from build123d import *

# Parameters (mm, degrees)
BOSS_EXTRUDE1_DEPTH = 1.6
SKETCH2_R           = 1.5875
CUT_EXTRUDE1_DEPTH  = 47.534935159


with BuildPart() as part:
    # Sketch1 → Boss-Extrude1 (new body)
    with BuildSketch(Plane(origin=(0, 0, 0), x_dir=(1, 0, 0), z_dir=(0, 1, 0))):
        with BuildLine():
            Line((-23.0632, 31.273950746), (-19.05, 31.273950746))
            ThreePointArc((-19.05, 31.273950746), (-15.214318255, 32.713055735), (-13.055721082, 36.195))
            Line((-13.055721082, 36.195), (-13.055721082, 40.386))
            Line((-13.055721082, 40.386), (13.055721082, 40.386))
            Line((13.055721082, 40.386), (13.055721082, 36.195))
            ThreePointArc((13.055721082, 36.195), (15.214318255, 32.713055735), (19.05, 31.273950746))
            Line((19.05, 31.273950746), (23.0632, 31.273950746))
            Line((23.0632, 31.273950746), (23.0632, -31.273950746))
            Line((23.0632, -31.273950746), (19.05, -31.273950746))
            ThreePointArc((19.05, -31.273950746), (15.214318255, -32.713055735), (13.055721082, -36.195))
            Line((13.055721082, -36.195), (13.055721082, -40.386))
            Line((13.055721082, -40.386), (-13.055721082, -40.386))
            Line((-13.055721082, -40.386), (-13.055721082, -36.195))
            ThreePointArc((-13.055721082, -36.195), (-15.214318255, -32.713055735), (-19.05, -31.273950746))
            Line((-19.05, -31.273950746), (-23.0632, -31.273950746))
            Line((-23.0632, -31.273950746), (-23.0632, 0))
            Line((-23.0632, 0), (-23.0632, 31.273950746))
        make_face()
    extrude(amount=BOSS_EXTRUDE1_DEPTH)

    # Sketch2 → Cut-Extrude1 (cut, through all)
    with BuildSketch(Plane(origin=(0, 1.6, 0), x_dir=(1, 0, 0), z_dir=(0, 1, 0))):
        with Locations(Location((-19.05, 12.7, 0), (0, 0, 270))):
            Circle(SKETCH2_R)
        with Locations(Location((19.05, 12.7, 0), (0, 0, 90))):
            Circle(SKETCH2_R)
        with Locations(Location((19.05, -12.7, 0), (0, 0, 270))):
            Circle(SKETCH2_R)
        with Locations(Location((-19.05, -12.7, 0), (0, 0, 90))):
            Circle(SKETCH2_R)
    extrude(amount=-CUT_EXTRUDE1_DEPTH, mode=Mode.SUBTRACT)


solid = part.part
The model under review builds one solid part; all positions refer to its coordinate system, in mm. A direction names the side the tool comes from. Coordinates: 2 decimals unless noted, no trailing zeros. Loops run counter-clockwise (first coordinate to the right, second up) from the corner with the lowest first, then second, coordinate; pieces in that order, holes last.
(1) Consider section A-A, the plane z = 12.7. Give the boundary of the cut face in (x, y), plus the area to 3 significant figures.
Determined:
outline: (-23.06, 0) - (-20.64, 0) - (-20.64, 1.6) - (-23.06, 1.6) - close; (-17.46, 0) - (17.46, 0) - (17.46, 1.6) - (-17.46, 1.6) - close; (20.64, 0) - (23.06, 0) - (23.06, 1.6) - (20.64, 1.6) - close
area: 63.6 mm2
(2) Insertion check: P1, Ø0.5, axis at x = -21, y = 1, coming from the -Z side; P2, Ø0.8, axis at y = 0.5, z = -39, coming from the +X side; P3, Ø0.5, axis at y = 1, z = -38.5, coming from the -X side. Each pin has a flat end and moves straight along its axis. Give the tip position at first contact, or say it passes through.
Determined:
P1: stops at z = -31.27
P2: stops at x = 13.06
P3: stops at x = -13.06
(3) Draft analysis for pull direction Z (two halves, no side actions). For faces 4 (the flat face through (-23.063, 1, 0)), 5 (the flat face through (-21, 1, -31.274)), 6 (the cylindrical face through (17.71, 0.81, -13.55)), state which applies: +Z half, -Z half, draft (parallel to the pull), parting line (faces both ways), or undercut.
Determined:
face 4: draft
face 5: -Z half
face 6: undercut
(4) Wall thickness on L1, parallel to X at y = 0.65, z = 12.7; L2, parallel to Z at x = 20, y = 1.15; L3, parallel to X at y = 0.9, z = 37: over which ranges is each line inside the solid? List them lowest first.
Determined:
L1: x = -23.06 to -20.64, -17.46 to 17.46, 20.64 to 23.06
L2: z = -31.27 to -13.97, -11.43 to 11.43, 13.97 to 31.27
L3: x = -13.06 to 13.06
(5) Consider section B-B, the plane y = 1.35. Give the number of separate pieces and of enclosed holes in the cut face, plus the area to 3 significant figures.
Determined:
separate pieces: 1
enclosed holes: 4
area: 3,360 mm2
(6) Tool access review of faces 1 (the flat face through (-13.056, 1, -38)), 2 (the flat face through (13.056, 1, -38)), 3 (the flat face through (-13.056, 1, 38)): name each direction out of +Z, -Z, +X, -X, +Y, -Y from which nothing blocks a thin tool from reaching the whole face with its end or side.
Determined:
face 1: -Z, -X, +Y, -Y
face 2: -Z, +X, +Y, -Y
face 3: +Z, -X, +Y, -Y
